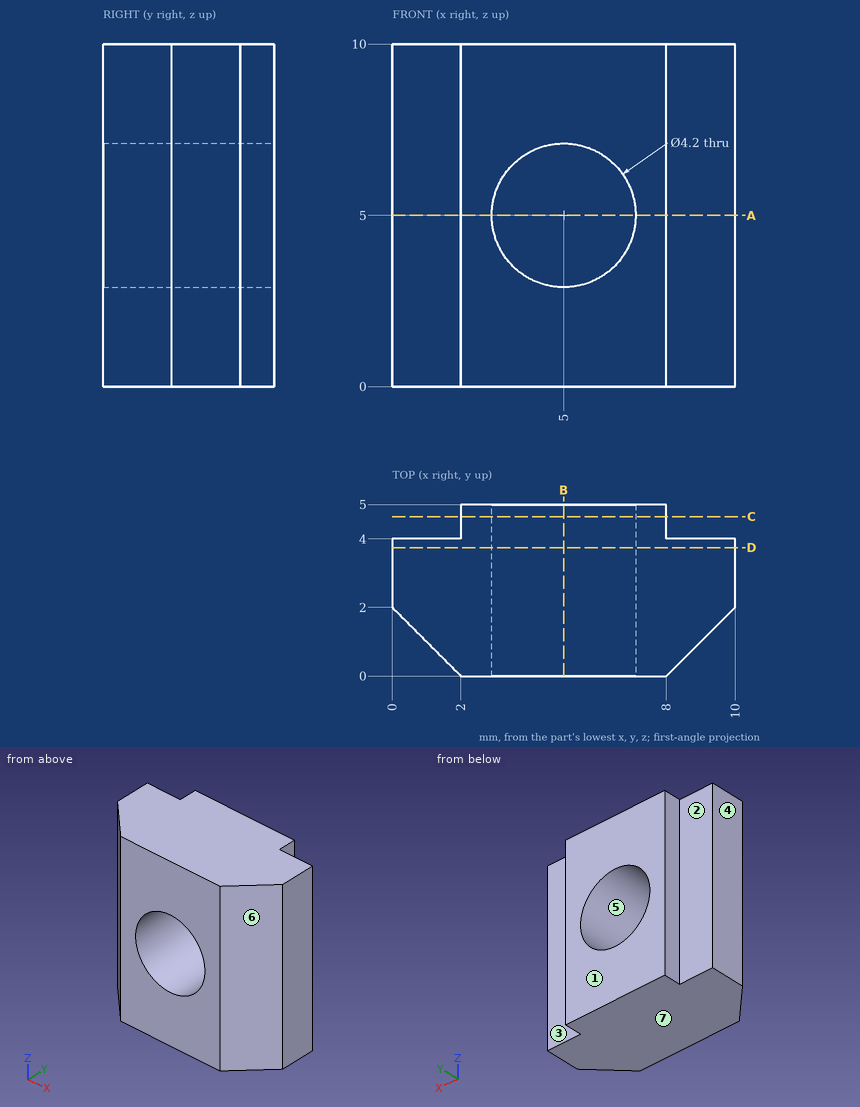
Geometry check sheet. Reference: drawing and pictorial views, mm from the part's lowest x, y, z. A direction names the side the tool comes from. Round coordinates to 2 decimals unless told otherwise and drop trailing zeros. Write each loop counter-clockwise with the first axis right and the second up, starting at its lowest first coordinate (ties: lowest second). Pieces come first, ordered by that corner, then holes.
Item 1: Section check C-C (y = 4.65). Record the boundary of the cut face in (x, z).
Determined:
outline: (2, 0) - (8, 0) - (8, 10) - (2, 10) - close; hole circle Ø4.2 at (5, 5)
Item 2: Section check D-D (y = 3.75). Record the boundary of the cut face in (x, z).
Determined:
outline: (0, 0) - (10, 0) - (10, 10) - (0, 10) - close; hole circle Ø4.2 at (5, 5)
Item 3: Go/stop test with flat-tipped pins: pin 1 Ø1 at (x, z) = (1, 4) entering from +Y; pin 2 Ø1 at (y, z) = (0.5, 9) entering from -X; pin 3 Ø0.5 at (y, z) = (4.5, 5) entering from -X. Record where each tip stops, or that it passes through.
Determined:
pin 1: stops at y = 4
pin 2: stops at x = 1
pin 3: stops at x = 2
Item 4: Section check A-A (z = 5). Record the boundary of the cut face in (x, y), plus the area to 3 significant figures.
Determined:
outline: (0, 2) - (2, 0) - (2.9, 0) - (2.9, 5) - (2, 5) - (2, 4) - (0, 4) - close; (7.1, 0) - (8, 0) - (10, 2) - (10, 4) - (8, 4) - (8, 5) - (7.1, 5) - close
area: 21.0 mm2
Item 5: Material ranges on line 1 along Z through (x, y) = (5, 2.45); line 2 along Z through (x, y) = (4.25, 2.5), recorded low to high.
Determined:
line 1: z = 0 to 2.9, 7.1 to 10
line 2: z = 0 to 3.04, 6.96 to 10
Item 6: Section check B-B (x = 5). Record the boundary of the cut face in (y, z).
Determined:
outline: (0, 0) - (5, 0) - (5, 2.9) - (0, 2.9) - close; (0, 7.1) - (5, 7.1) - (5, 10) - (0, 10) - close
Item 7: Access from +Z, -Z, +X, -X, +Y, -Y to the whole of each face (thin tool, end or side, straight path). Record for the marked faces 1, 2 and 3.
Determined:
face 1: +Z, -Z, +X, -X, +Y
face 2: +Z, -Z, -X, +Y
face 3: +Z, -Z, +X, +Y
Item 8: Mould release check, pull along X, two halves, no side actions. Record for the marked faces 4, 5, 6 and 7: +X half, -X half, draft (parallel to the pull), parting line (faces both ways), or undercut.
Determined:
face 4: -X half
face 5: undercut
face 6: +X half
face 7: draft
